Verification items for the finished model (mm, model axes). A direction names the side the tool comes from. Coordinates: 2 decimals unless noted, no trailing zeros. Write each loop counter-clockwise with the first axis right and the second up, starting at its lowest first coordinate (ties: lowest second). Pieces come first, ordered by that corner, then holes. Notation, with made-up numbers: M 44,-14 L 67,-14 A29 cw 67,21 Z; hole C 79,82 d8. An arc over 180 degrees is marked long. Answer in a Markdown table with one row per item.
Autodesk Inventor part; units mm, degrees
ref_plane "Work Plane1" through (0, 5, 0) normal (0, 1, 0) x (1, 0, 0)
ref_plane "YZ Plane" through (0, 0, 0) normal (1, 0, 0) x (0, 1, 0)
ref_plane "XZ Plane" through (0, 0, 0) normal (0, 1, 0) x (-1, 0, 0)
sketch "Sketch2" plane through (0, 0, 0) normal (0, 1, 0) x (-1, 0, 0)
  circle A0 centre (0, 0) radius 45 construction
  arc A1 (35.8767, 27.1636) -> (35.8767, -27.1636) centre (73, 0) ccw
  arc A2 (-27.1636, 35.8767) -> (27.1636, 35.8767) centre (0, 73) ccw
  arc A3 (-35.8767, -27.1636) -> (-35.8767, 27.1636) centre (-73, 0) ccw
  arc A4 (27.1636, -35.8767) -> (-27.1636, -35.8767) centre (0, -73) ccw
  circle A5 centre (0, 0) radius 20 construction
  line L0 (0, 0) -> (31.8198, -31.8198) construction
  line L1 (0, 0) -> (45, 0) construction
  arc A6 (16.7584, -11.5258) -> (11.5258, -16.7584) centre (14.1421, -14.1421) ccw
  line L2 (16.7584, -11.5258) -> (34.3284, -29.0958)
  line L3 (11.5258, -16.7584) -> (29.0958, -34.3284)
  arc A7 (34.3284, -29.0958) -> (35.8767, -27.1636) centre (0, 0) ccw
  arc A8 (27.1636, -35.8767) -> (29.0958, -34.3284) centre (0, 0) ccw
  arc A9 (11.5258, 16.7584) -> (16.7584, 11.5258) centre (14.1421, 14.1421) ccw
  line L4 (16.7584, 11.5258) -> (34.3284, 29.0958)
  line L5 (11.5258, 16.7584) -> (29.0958, 34.3284)
  arc A10 (29.0958, 34.3284) -> (27.1636, 35.8767) centre (0, 0) ccw
  arc A11 (35.8767, 27.1636) -> (34.3284, 29.0958) centre (0, 0) ccw
  arc A12 (-16.7584, 11.5258) -> (-11.5258, 16.7584) centre (-14.1421, 14.1421) ccw
  line L6 (-11.5258, 16.7584) -> (-29.0958, 34.3284)
  line L7 (-16.7584, 11.5258) -> (-34.3284, 29.0958)
  arc A13 (-34.3284, 29.0958) -> (-35.8767, 27.1636) centre (0, 0) ccw
  arc A14 (-27.1636, 35.8767) -> (-29.0958, 34.3284) centre (0, 0) ccw
  arc A15 (-11.5258, -16.7584) -> (-16.7584, -11.5258) centre (-14.1421, -14.1421) ccw
  line L8 (-16.7584, -11.5258) -> (-34.3284, -29.0958)
  line L9 (-11.5258, -16.7584) -> (-29.0958, -34.3284)
  arc A16 (-29.0958, -34.3284) -> (-27.1636, -35.8767) centre (0, 0) ccw
  arc A17 (-35.8767, -27.1636) -> (-34.3284, -29.0958) centre (0, 0) ccw
  point P0 (27.1636, 35.8767)
  point P1 (-27.1636, 35.8767)
  point P2 (-35.8767, 27.1636)
  point P3 (-27.1636, -35.8767)
  point P4 (35.8767, 27.1636)
  dimension "d14" = 40
  dimension "d7" = 90
  dimension "d8" = 46
  dimension "d9" = 73
  dimension "d12" = 360
  dimension "d15" = 45
  dimension "d16" = 7.4
  dimension "d19" = 360
extrude "Extrusion1" add sketch "Sketch2" along normal blind 10
sketch "Sketch3" plane through (0, 10, 0) normal (0, 1, 0) x (1, 0, 0)
  arc A0 (27.1636, -35.8767) -> (-27.1636, -35.8767) centre (0, -73) ccw
  line L0 (29.0958, -34.3284) -> (11.5258, -16.7584)
  arc A1 (16.7584, -11.5258) -> (11.5258, -16.7584) centre (14.1421, -14.1421) ccw
  line L1 (16.7584, -11.5258) -> (34.3284, -29.0958)
  arc A2 (35.8767, 27.1636) -> (35.8767, -27.1636) centre (73, 0) ccw
  line L2 (34.3284, 29.0958) -> (16.7584, 11.5258)
  arc A3 (11.5258, 16.7584) -> (16.7584, 11.5258) centre (14.1421, 14.1421) ccw
  line L3 (11.5258, 16.7584) -> (29.0958, 34.3284)
  arc A4 (-27.1636, 35.8767) -> (27.1636, 35.8767) centre (0, 73) ccw
  line L4 (-29.0958, 34.3284) -> (-11.5258, 16.7584)
  arc A5 (-16.7584, 11.5258) -> (-11.5258, 16.7584) centre (-14.1421, 14.1421) ccw
  line L5 (-16.7584, 11.5258) -> (-34.3284, 29.0958)
  arc A6 (-35.8767, -27.1636) -> (-35.8767, 27.1636) centre (-73, 0) ccw
  line L6 (-34.3284, -29.0958) -> (-16.7584, -11.5258)
  arc A7 (-11.5258, -16.7584) -> (-16.7584, -11.5258) centre (-14.1421, -14.1421) ccw
  line L7 (-11.5258, -16.7584) -> (-29.0958, -34.3284)
  line L8 (-15.5707, -23.6317) -> (-10.1116, -18.1726)
  arc A8 (-10.1116, -18.1726) -> (-18.1726, -10.1116) centre (-14.1421, -14.1421) ccw
  line L9 (-18.1726, -10.1116) -> (-23.6317, -15.5707)
  arc A9 (-26.9641, -13.5902) -> (-26.9641, 13.5902) centre (-73, 0) ccw
  line L10 (-23.6317, 15.5707) -> (-18.1726, 10.1116)
  arc A10 (-18.1726, 10.1116) -> (-10.1116, 18.1726) centre (-14.1421, 14.1421) ccw
  line L11 (-10.1116, 18.1726) -> (-15.5707, 23.6317)
  arc A11 (-13.5902, 26.9641) -> (13.5902, 26.9641) centre (0, 73) ccw
  line L12 (15.5707, 23.6317) -> (10.1116, 18.1726)
  arc A12 (10.1116, 18.1726) -> (18.1726, 10.1116) centre (14.1421, 14.1421) ccw
  line L13 (18.1726, 10.1116) -> (23.6317, 15.5707)
  arc A13 (26.9641, 13.5902) -> (26.9641, -13.5902) centre (73, 0) ccw
  line L14 (23.6317, -15.5707) -> (18.1726, -10.1116)
  arc A14 (18.1726, -10.1116) -> (10.1116, -18.1726) centre (14.1421, -14.1421) ccw
  line L15 (10.1116, -18.1726) -> (15.5707, -23.6317)
  arc A15 (13.5902, -26.9641) -> (-13.5902, -26.9641) centre (0, -73) ccw
  arc A16 (-15.5707, -23.6317) -> (-13.5902, -26.9641) centre (-14.1565, -25.0459) ccw
  arc A17 (-26.9641, -13.5902) -> (-23.6317, -15.5707) centre (-25.0459, -14.1565) ccw
  arc A18 (-23.6317, 15.5707) -> (-26.9641, 13.5902) centre (-25.0459, 14.1565) ccw
  arc A19 (-13.5902, 26.9641) -> (-15.5707, 23.6317) centre (-14.1565, 25.0459) ccw
  arc A20 (15.5707, 23.6317) -> (13.5902, 26.9641) centre (14.1565, 25.0459) ccw
  arc A21 (26.9641, 13.5902) -> (23.6317, 15.5707) centre (25.0459, 14.1565) ccw
  arc A22 (23.6317, -15.5707) -> (26.9641, -13.5902) centre (25.0459, -14.1565) ccw
  arc A23 (13.5902, -26.9641) -> (15.5707, -23.6317) centre (14.1565, -25.0459) ccw
  point P0 (-22.5835, -30.6446)
  point P1 (-30.6446, -22.5835)
  point P2 (-30.6446, 22.5835)
  point P3 (-22.5835, 30.6446)
  point P4 (22.5835, 30.6446)
  point P5 (30.6446, 22.5835)
  point P6 (30.6446, -22.5835)
  point P7 (22.5835, -30.6446)
  dimension "d23" = 2
  dimension "d24" = 2
extrude "Extrusion2" cut sketch "Sketch3" against normal blind 0.5
ref_plane "Work Plane1" through (0, 5, 0) normal (0, 1, 0) x (1, 0, 0)
mirror "Mirror1" about plane through (0, 5, 0) normal (0, 1, 0) of "Extrusion2"
sketch "Sketch4" plane through (0, 9.5, 0) normal (0, 1, 0) x (1, 0, 0)
  circle A0 centre (0, 0) radius 9
  dimension "d27" = 18
extrude "Extrusion3" add sketch "Sketch4" along normal blind 10
sketch "Sketch5" plane through (0, 19.5, 0) normal (0, 1, 0) x (1, 0, 0)
  circle A0 centre (0, 0) radius 9
hole "Hole1" at (0, 19.5, 0) direction (0, -1, 0) diameter 9 end through all
chamfer "Chamfer1" distance 1 angle 45 1 edges at (-9, 19.5, 0)
fillet "Fillet1" radius 2 1 edges at (-9, 9.5, 0)
chamfer "Chamfer3" distance 0.5 angle 45 8 edges at (-27, 10, 0) (0, 10, -27) (27, 10, 0) (0, 10, 27) (0, 0, 27) (-27, 0, 0) (0, 0, -27) (27, 0, 0)
properties part number "Malta cross"
1) Thickness scan on L1, parallel to Z at x = 0, y = 7.5; L2, parallel to X at y = 4.5, z = -19. Record the ranges inside material, lowest first. Write a range as [from, to].
Response values:
| item | result |
|---|---|
| L1 | z = [-27, -4.5], [4.5, 27] |
| L2 | x = [-31.11, -24.23], [-13.77, 13.77], [24.23, 31.11] |
2) Release check for a two-part mould opening along X. For faces 1 (the face through (10.024, 0.246, 10.201)), 2 (the face through (-10, 0, -13)), 3 (the face through (-35.127, 4.93, -28.127)) record: +X half, -X half, draft (parallel to the pull), parting line (faces both ways), or undercut.
Response values:
| item | result |
|---|---|
| face 1 | undercut |
| face 2 | draft |
| face 3 | -X half |
3) Sectioned sample at B-B (y = 5.75). Record the cut outline in (x, z).
Response values:
| item | result |
|---|---|
| outline | M -35.88,-27.16 A44.91 ccw -34.33,-29.1 L -16.76,-11.53 A3.7 cw -11.53,-16.76 L -29.1,-34.33 A45.09 ccw -27.16,-35.88 A46 cw 27.16,-35.88 A44.91 ccw 29.1,-34.33 L 11.53,-16.76 A3.7 cw 16.76,-11.53 L 34.33,-29.1 A45.09 ccw 35.88,-27.16 A46 cw 35.88,27.16 A44.91 ccw 34.33,29.1 L 16.76,11.53 A3.7 cw 11.53,16.76 L 29.1,34.33 A45.09 ccw 27.16,35.88 A46 cw -27.16,35.88 A44.91 ccw -29.1,34.33 L -11.53,16.76 A3.7 cw -16.76,11.53 L -34.33,29.1 A45.09 ccw -35.88,27.16 A46 cw Z; hole C 0,0 d9 |
4) Sectioned sample at C-C (x = 0). Record the cut outline in (y, z).
Response values:
| item | result |
|---|---|
| outline | M 0,-26.5 L 0.5,-27 L 9.5,-27 L 10,-26.5 L 10,-25 L 9.5,-25 L 9.5,-11 A2 cw 11.5,-9 L 18.5,-9 L 19.5,-8 L 19.5,-4.5 L 0.5,-4.5 L 0.5,-25 L 0,-25 Z; M 0,25 L 0.5,25 L 0.5,4.5 L 19.5,4.5 L 19.5,8 L 18.5,9 L 11.5,9 A2 cw 9.5,11 L 9.5,25 L 10,25 L 10,26.5 L 9.5,27 L 0.5,27 L 0,26.5 Z |
5) Tool access check on faces 4 (the face through (-20.94, 0.25, 12.88)), 5 (the face through (26.86, 0.36, 0.41)), 6 (the face through (12.88, 9.75, -20.94)). Record the directions out of +Z, -Z, +X, -X, +Y, -Y that give a thin tool (end or side, any length) a straight path to the whole face; none if there is none.
Response values:
| item | result |
|---|---|
| face 4 | -Y |
| face 5 | +X, -Y |
| face 6 | +Y |
6) Sectioned sample at D-D (x = -20.5). Give the number of separate pieces and of enclosed holes in the cut face, then the cut area to 3 significant figures.
Response values:
| item | result |
|---|---|
| separate pieces | 3 |
| enclosed holes | 0 |
| area | 402 mm² |
7) Sectioned sample at A-A (z = 0). Record the cut outline in (x, y), then the cut area to 3 significant figures.
Response values:
| item | result |
|---|---|
| outline | M -27,0.5 L -26.5,0 L -25,0 L -25,0.5 L -4.5,0.5 L -4.5,19.5 L -8,19.5 L -9,18.5 L -9,11.5 A2 cw -11,9.5 L -25,9.5 L -25,10 L -26.5,10 L -27,9.5 Z; M 4.5,0.5 L 25,0.5 L 25,0 L 26.5,0 L 27,0.5 L 27,9.5 L 26.5,10 L 25,10 L 25,9.5 L 11,9.5 A2 cw 9,11.5 L 9,18.5 L 8,19.5 L 4.5,19.5 Z |
| area | 499 mm² |
8) Depth check by flat-ended pin: pin 1 (8 mm diameter, centred on x = -3.5, z = 17.5, fed in from +Y); pin 2 (6 mm diameter, centred on y = 3, z = -9.5, fed in from +X); pin 3 (6 mm diameter, centred on x = -21, y = 3.5, fed in from +Z). Enter the tip coordinate at first touch or a pass-through.
Response values:
| item | result |
|---|---|
| pin 1 | stops at y = 9.5 |
| pin 2 | stops at x = 28.73 |
| pin 3 | stops at z = 33.76 |
